```python
from build123d import *

# Parameters (mm, degrees)
F0_R     = 1.02362
F0_R_2   = 1.5875
F1_DEPTH = 1.5875
F2_SIZE2 = 0.762
F2_SIZE  = 0.762


with BuildPart() as f1:
    # F0 (on Front) → F1 (new body, symmetric)
    with BuildSketch(Plane.XZ):
        with BuildLine():
            Line((-4.501804, -1.775407), (-4.471419, -3.052185))
            ThreePointArc((-4.471419, -3.052185), (-2.092182, -4.085642), (0.47765, -4.438859))
            Line((0.47765, -4.438859), (0.47765, -2.851359))
            Line((0.47765, -2.851359), (5.742792, -2.851359))
            ThreePointArc((5.742792, -2.851359), (1.310194, 14.574686), (-6.089304, -1.813188))
            Line((-6.089304, -1.813188), (-4.501804, -1.775407))
        make_face()
        with Locations((7.089037, 2.107543)):
            Circle(F0_R, mode=Mode.SUBTRACT)
        with Locations((0.47765, 5.086141)):
            Circle(F0_R_2, mode=Mode.SUBTRACT)
    extrude(amount=F1_DEPTH, both=True)

    # F2
    f2_edges = [f1.edges().sort_by_distance(p)[0] for p in [
        (6.065417, -1.5875, 2.107543),
    ]]
    chamfer(f2_edges, length=F2_SIZE, length2=F2_SIZE2)


solid = f1.part
```
Input: part model. Units: mm. Frame: model coordinates. A direction names the side the tool comes from. Round coordinates to 2 decimals unless told otherwise and drop trailing zeros. Loops run counter-clockwise (first coordinate to the right, second up) from the corner with the lowest first, then second, coordinate; pieces in that order, holes last. Notation, with made-up numbers: (81, 63.25) -> (122, 63.25) arc R7 cw to (122, 70.25) -> close; hole circle Ø2 at (70, 68.25). An arc over 180 degrees is marked (long way). Use one line per item in the form item = value. Start each with the question number.
Item 1: Set-up query: faces 4 (the face through (3, 0, -2.851)), 5 (the face through (-2.127, -0.022, -4.076)). Return all of +Z, -Z, +X, -X, +Y, -Y with unobstructed straight access to the full face (end or side cutting, diameter ignored); none if empty.
Item 2: Contact query for a flat-ended pin moving along its axis: pin 1 Ø1.6 at (x, z) = (7.09, 2.11) entering from +Y. Output: stop coordinate, or through.
Item 3: Section query B-B on z = 4.5. Return the cut outline in (x, y).
Item 4: Section query A-A on x = 1. Return the cut outline in (y, z), then the cut area to 3 significant figures.
Item 5: Mould query, pull axis Z, two halves, no side actions, for faces 1 (the face through (6.335, 0.398, 2.799)), 2 (the face through (0, -1.588, 7)), 3 (the face through (1.64, -0.02, 14.54)). Classes: pulls with the +Z half, pulls with the -Z half, needs draft (parallel to the pull), parting line crosses it, or undercut.
Item 6: Section query C-C on y = -1.05. Count the separate pieces of the cut face and the enclosed holes in it, then the cut area to 3 significant figures.
Item 7: Section query D-D on z = -0.5. Return the cut outline in (x, y), then the cut area to 3 significant figures.
Item 8: Material intervals for L1, parallel to X at y = 0.35, z = 1.5; L2, parallel to X at y = 0, z = 4.25; L3, parallel to Z at x = -0.25, y = -0.7, sorted ascending. Write a range as from..to.
Ans:
q1.face_4 = -Z, +X, +Y, -Y
q1.face_5 = -Z, -X, +Y, -Y
q2.pin_1 = through
q3.outline = (-9.03, -1.59) -> (-1, -1.59) -> (-1, 1.59) -> (-9.03, 1.59) -> close; (1.95, -1.59) -> (9.98, -1.59) -> (9.98, 1.59) -> (1.95, 1.59) -> close
q4.outline = (-1.59, -2.85) -> (1.59, -2.85) -> (1.59, 3.59) -> (-1.59, 3.59) -> close; (-1.59, 6.59) -> (1.59, 6.59) -> (1.59, 14.6) -> (-1.59, 14.6) -> close
q4.area = 45.9 mm^2
q5.face_1 = undercut
q5.face_2 = needs draft
q5.face_3 = parting line crosses it
q6.separate_pieces = 1
q6.enclosed_holes = 2
q6.area = 265 mm^2
q7.outline = (-7.24, -1.59) -> (8.19, -1.59) -> (8.19, 1.59) -> (-7.24, 1.59) -> close
q7.area = 49.0 mm^2
q8.L1 = -8.35..6.27, 7.91..9.3
q8.L2 = -9.01..-0.87, 1.83..9.97
q8.L3 = -4.41..3.68, 6.5..14.58
